from build123d import *

# Parameters (mm, degrees)
SKETCH1_R           = 4.0386
BOSS_EXTRUDE1_DEPTH = 2.54
SKETCH1_4_R         = 10.9855
SKETCH1_4_R_2       = 4.0386
BOSS_EXTRUDE2_DEPTH = 3.81
FILLET1_R           = 2.54
FILLET2_R           = 12.7
SKETCH1_6_R         = 4.0386
BOSS_EXTRUDE3_DEPTH = 2.54
SKETCH3_R           = 2.54
BOSS_EXTRUDE4_DEPTH = 3.81


with BuildPart() as part:
    # Sketch1 → Boss-Extrude1 (new body)
    with BuildSketch(Plane.XY):
        Circle(SKETCH1_R)
    extrude(amount=BOSS_EXTRUDE1_DEPTH)

    # Sketch1<4> → Boss-Extrude2 (add)
    with BuildSketch(Plane.XY):
        with Locations(Location((0, 0, 0), (0, 0, 180))):
            Circle(SKETCH1_4_R)
        with Locations(Location((0, 0, 0), (0, 0, 180))):
            Circle(SKETCH1_4_R_2, mode=Mode.SUBTRACT)
    extrude(amount=BOSS_EXTRUDE2_DEPTH)

    # Fillet1
    # the kernel refuses this fillet: 2.54 mm, written as the material it takes off along each edge
    with BuildSketch(Plane(origin=(0, 0, 3.81), x_dir=(-1, 0, 0), z_dir=(0, 1, 0))) as fillet1_piece_1:
        with BuildLine():
            CenterArc((6.238304526, -2.54), FILLET1_R, 90, 60)
            Line((4.0386, -1.27), (3.994605909, -1.2446))
            ThreePointArc((3.994605909, -1.2446), (3.9878, -0.635), (3.9878, 0))
            Line((3.9878, 0), (4.0386, 0.0508))
            Line((4.0386, 0.0508), (6.238304526, 0.0508))
            Line((6.238304526, 0.0508), (6.238304526, 0))
        make_face()
    revolve(axis=Axis((0, 0, 3.81), (0, 0, 1)), mode=Mode.SUBTRACT)

    # Fillet2
    fillet2_edges = [part.edges().sort_by_distance(p)[0] for p in [
        (4.0386, 0, 2.54),
    ]]
    fillet(fillet2_edges, radius=FILLET2_R)

    # Sketch1<6> → Boss-Extrude3 (add)
    with BuildSketch(Plane.XY):
        Circle(SKETCH1_6_R)
    extrude(amount=-BOSS_EXTRUDE3_DEPTH)

    # Sketch3 → Boss-Extrude4 (add)
    with BuildSketch(Plane(origin=(0, 0, -2.54), x_dir=(-1, 0, 0), z_dir=(0, 0, -1))):
        with Locations(Location((0, 0, 0), (0, 0, 180))):
            Circle(SKETCH3_R)
    extrude(amount=BOSS_EXTRUDE4_DEPTH)


solid = part.part
Model file for the job. Use its own axes, mm. A direction names the side the tool comes from. Give positions to 0.01 mm unless a question says otherwise; leave off trailing zeros. Loops run counter-clockwise (first coordinate to the right, second up) from the corner with the lowest first, then second, coordinate; pieces in that order, holes last.
1) Saw through at C-C (z = -3.25). Write the cut outline in (x, y).
2) Tool access for faces 1 (the flat face through (0, 0, -6.35)), 2 (the flat face through (0, -3, -2.54)): list every direction of +Z, -Z, +X, -X, +Y, -Y with a clear straight run to the whole face (end or side of a thin tool).
3) Saw through at A-A (z = -1). Write the cut outline in (x, y).
4) Saw through at B-B (y = -9.25). Write the cut outline in (x, z), plus the area to 3 significant figures.
5) Wall check: line 1 (Z direction, x = -8.75, y = 6.5); line 2 (Y direction, x = 3.5, z = -0.5); line 3 (Y direction, x = 2.5, z = -0.75). Give the ranges that are in metal, low to high.
6) Flat gauge pins, fed straight in: pin 1 Ø5 at (x, y) = (-8, -3) entering from -Z; pin 2 Ø1 at (x, z) = (0.5, -3.5) entering from +Y; pin 3 Ø4 at (y, z) = (2.5, 2) entering from +X. Where does each tip first touch, or does it go through?
Answer block:
1. outline: circle Ø5.08 at (0, 0)
2. face 1: -Z, +X, -X, +Y, -Y
2. face 2: -Z
3. outline: circle Ø8.08 at (0, 0)
4. outline: (-5.93, 0) - (5.93, 0) - (5.93, 3.81) - (-5.93, 3.81) - close
4. area: 45.2 mm2
5. line 1: z = 0 to 3.81
5. line 2: y = -2.02 to 2.02
5. line 3: y = -3.17 to 3.17
6. pin 1: stops at z = 0
6. pin 2: stops at y = 2.54
6. pin 3: stops at x = 10.97
